Source: CAD feature listing. Evaluate the final solid. Frame: model axes, mm. A direction names the side the tool comes from. Coordinates: 2 decimals unless noted, no trailing zeros. Order: outer loops, then holes, each group sorted by start corner. A loop starts at its lowest first (then second) coordinate and runs counter-clockwise, first axis right, second up. Notation, with made-up numbers: (10, 83.25) - (17, 83.25) arc R20 ccw to (17, 116.25) - close; hole circle Ø3 at (-8.5, -2.75). An arc over 180 degrees is marked (long way). One line per question, with ' | ' between items. Start each with the question number.
(1) Contact query for flat-ended pins moving along their axis: P1, Ø2, axis at x = 17, z = -33.5, coming from the +Y side; P2, Ø4.5, axis at x = 340, z = -87.5, coming from the +Y side; P3, Ø4.5, axis at x = -342.5, z = -81.5, coming from the -Y side. Output: stop coordinate, or through.
(2) Draft query along X for faces 5 (the flat face through (350, -18, -9)), 6 (the flat face through (-141, -30, -1)), 7 (the flat face through (-344, 2.5, -85)), 8 (the conical face through (43.686, -10.906, -13.757)). Return one class per face: +X half, -X half, draft (parallel to the pull), parting line (faces both ways), or undercut.
(3) Section A-A (x = 280). Return the cut outline in (y, z).
(4) Access query for faces 1 (the flat face through (344, 2.5, -85)), 2 (the flat face through (279, -30, -1)), 3 (the flat face through (344, 17.5, -85)), 4 (the flat face through (-5, -57.8, -1)). Directions: +Z, -Z, +X, -X, +Y, -Y. A direction counts if a zero-diameter tool reaches every point of the face in a straight line with its end or side. Return the directions, or none.
(5) Section B-B (y = -17). Return the cut outline in (x, z).
(6) Line query: line 1 along X through (y, z) = (15.5, 30); line 2 along Z through (x, y) = (93, -40.5); line 3 along Y through (x, z) = (275.5, 16.5). Output: solid intervals per line, ascending.
from build123d import *

# Parameters (mm, degrees)
SKETCH1_W                = 700
SKETCH1_H                = 150
BOSS_EXTRUDE1_DEPTH      = 20
BOSS_EXTRUDE1_DEPTH_BACK = 57.8
SKETCH3_W                = 15
SKETCH3_H                = 15
BOSS_EXTRUDE2_DEPTH      = 20
CUT_EXTRUDE1_DEPTH       = 15
CUT_EXTRUDE2_DEPTH       = 15
SKETCH6_R                = 51.25
CUT_EXTRUDE3_DEPTH       = 50
CUT_EXTRUDE3_TAPER       = 10
SKETCH7_R                = 51.25
CUT_EXTRUDE4_DEPTH       = 50
CUT_EXTRUDE4_TAPER       = 10
SKETCH8_R                = 51.25
CUT_EXTRUDE5_DEPTH       = 50
CUT_EXTRUDE5_TAPER       = 10
SKETCH9_R                = 51.25
CUT_EXTRUDE6_DEPTH       = 50
CUT_EXTRUDE6_TAPER       = 10
SKETCH10_R               = 51.25
CUT_EXTRUDE7_DEPTH       = 50
CUT_EXTRUDE7_TAPER       = 10


with BuildPart() as part:
    # Sketch1 → Boss-Extrude1 (new body, two sides)
    with BuildSketch(Plane(origin=(0, 0, 0), x_dir=(1, 0, 0), z_dir=(0, 1, 0))) as boss_extrude1_sk:
        Rectangle(SKETCH1_W, SKETCH1_H)
    extrude(amount=BOSS_EXTRUDE1_DEPTH)
    extrude(boss_extrude1_sk.sketch, amount=-BOSS_EXTRUDE1_DEPTH_BACK)

    # Sketch3 → Boss-Extrude2 (add)
    with BuildSketch(Plane(origin=(0, 0, -75), x_dir=(-1, 0, 0), z_dir=(0, 0, -1))):
        with Locations((-342.5, 10)):
            Rectangle(SKETCH3_W, SKETCH3_H)
        with Locations((342.5, 10)):
            Rectangle(SKETCH3_W, SKETCH3_H)
    extrude(amount=BOSS_EXTRUDE2_DEPTH)

    # Sketch4 → Cut-Extrude1 (cut)
    with BuildSketch(Plane(origin=(0, 17.5, 0), x_dir=(1, 0, 0), z_dir=(0, 1, 0))):
        Polygon((340, 90), (335, 90), (335, 85), align=None)
        Polygon((340, 85), (335, 85), (335, 80), align=None)
        Polygon((335, 95), (335, 90), (340, 95), align=None)
    extrude(amount=-CUT_EXTRUDE1_DEPTH, mode=Mode.SUBTRACT)

    # Sketch5 → Cut-Extrude2 (cut)
    with BuildSketch(Plane(origin=(0, 17.5, 0), x_dir=(1, 0, 0), z_dir=(0, 1, 0))):
        Polygon((-335, 85), (-335, 90), (-340, 90), align=None)
        Polygon((-335, 90), (-335, 95), (-340, 95), align=None)
        Polygon((-335, 80), (-335, 85), (-340, 85), align=None)
    extrude(amount=-CUT_EXTRUDE2_DEPTH, mode=Mode.SUBTRACT)

    # Sketch6 → Cut-Extrude3 (cut)
    with BuildSketch(Plane(origin=(0, 20, 0), x_dir=(1, 0, 0), z_dir=(0, 1, 0))):
        Circle(SKETCH6_R)
    extrude(amount=-CUT_EXTRUDE3_DEPTH, taper=CUT_EXTRUDE3_TAPER, mode=Mode.SUBTRACT)

    # Sketch7 → Cut-Extrude4 (cut)
    with BuildSketch(Plane(origin=(0, 20, 0), x_dir=(1, 0, 0), z_dir=(0, 1, 0))):
        with Locations((140, 0)):
            Circle(SKETCH7_R)
    extrude(amount=-CUT_EXTRUDE4_DEPTH, taper=CUT_EXTRUDE4_TAPER, mode=Mode.SUBTRACT)

    # Sketch8 → Cut-Extrude5 (cut)
    with BuildSketch(Plane(origin=(0, 20, 0), x_dir=(1, 0, 0), z_dir=(0, 1, 0))):
        with Locations((280, 0)):
            Circle(SKETCH8_R)
    extrude(amount=-CUT_EXTRUDE5_DEPTH, taper=CUT_EXTRUDE5_TAPER, mode=Mode.SUBTRACT)

    # Sketch9 → Cut-Extrude6 (cut)
    with BuildSketch(Plane(origin=(0, 20, 0), x_dir=(1, 0, 0), z_dir=(0, 1, 0))):
        with Locations((-140, 0)):
            Circle(SKETCH9_R)
    extrude(amount=-CUT_EXTRUDE6_DEPTH, taper=CUT_EXTRUDE6_TAPER, mode=Mode.SUBTRACT)

    # Sketch10 → Cut-Extrude7 (cut)
    with BuildSketch(Plane(origin=(0, 20, 0), x_dir=(1, 0, 0), z_dir=(0, 1, 0))):
        with Locations((-280, 0)):
            Circle(SKETCH10_R)
    extrude(amount=-CUT_EXTRUDE7_DEPTH, taper=CUT_EXTRUDE7_TAPER, mode=Mode.SUBTRACT)


solid = part.part
Response values:
1) P1: stops at y = -30 | P2: stops at y = 17.5 | P3: stops at y = 2.5
2) face 5: +X half | face 6: undercut | face 7: draft | face 8: undercut
3) outline: (-57.8, -75) - (20, -75) - (20, -51.25) - (-30, -42.43) - (-30, 42.43) - (20, 51.25) - (20, 75) - (-57.8, 75) - close
4) face 1: -Z, +X, -X, -Y | face 2: +Y | face 3: -Z, +X, -X, +Y | face 4: +Z, -Z, +X, -X, -Y
5) outline: (-350, -75) - (350, -75) - (350, 75) - (-350, 75) - close; hole circle Ø89.45 at (-280, 0); hole circle Ø89.45 at (-140, 0); hole circle Ø89.45 at (0, 0); hole circle Ø89.45 at (140, 0); hole circle Ø89.45 at (280, 0)
6) line 1: x = -350 to -320.57, -239.43 to -180.57, -99.43 to -40.57, 40.57 to 99.43, 180.57 to 239.43, 320.57 to 350 | line 2: z = -75 to 75 | line 3: y = -57.8 to -30
